```python
from build123d import *

# Parameters (mm, degrees)
SKETCH1_W           = 58
SKETCH1_H           = 23
BOSS_EXTRUDE1_DEPTH = 3
SKETCH2_W           = 3
SKETCH2_H           = 23
BOSS_EXTRUDE2_DEPTH = 1.5
SKETCH3_R           = 0.375
BOSS_EXTRUDE3_DEPTH = 5
LPATTERN1_COUNT     = 2
LPATTERN1_PITCH     = 50.8
SKETCH4_R           = 0.375
BOSS_EXTRUDE4_DEPTH = 5


with BuildPart() as part:
    # Sketch1 → Boss-Extrude1 (new body)
    with BuildSketch(Plane(origin=(0, 0, 0), x_dir=(1, 0, 0), z_dir=(0, 1, 0))):
        Rectangle(SKETCH1_W, SKETCH1_H)
    extrude(amount=BOSS_EXTRUDE1_DEPTH)

    # Sketch2 → Boss-Extrude2 (add)
    with BuildSketch(Plane.XZ):
        with Locations((-25.5, 0)):
            Rectangle(SKETCH2_W, SKETCH2_H)
    boss_extrude2 = extrude(amount=BOSS_EXTRUDE2_DEPTH)

    # Sketch3 → Boss-Extrude3 (add)
    with BuildSketch(Plane.XZ.offset(1.5)):
        with Locations(Location((-25.5, 8, 0), (0, 0, 270))):
            Circle(SKETCH3_R)
        with Locations(Location((-25.5, 0, 0), (0, 0, 270))):
            Circle(SKETCH3_R)
        with Locations(Location((-25.5, -8, 0), (0, 0, 270))):
            Circle(SKETCH3_R)
    extrude(amount=BOSS_EXTRUDE3_DEPTH)

    # LPattern1: Boss-Extrude2 ×2
    with Locations(*[(i * LPATTERN1_PITCH, 0, 0) for i in range(1, LPATTERN1_COUNT)]):
        add(boss_extrude2)

    # Sketch4 → Boss-Extrude4 (add)
    with BuildSketch(Plane.XZ.offset(1.5)):
        with Locations(Location((25.3, 8.5, 0), (0, 0, 270))):
            Circle(SKETCH4_R)
        with Locations(Location((25.3, 4.25, 0), (0, 0, 270))):
            Circle(SKETCH4_R)
        with Locations(Location((25.3, 0, 0), (0, 0, 270))):
            Circle(SKETCH4_R)
        with Locations(Location((25.3, -4.25, 0), (0, 0, 270))):
            Circle(SKETCH4_R)
        with Locations(Location((25.3, -8.5, 0), (0, 0, 270))):
            Circle(SKETCH4_R)
    extrude(amount=BOSS_EXTRUDE4_DEPTH)


solid = part.part
```
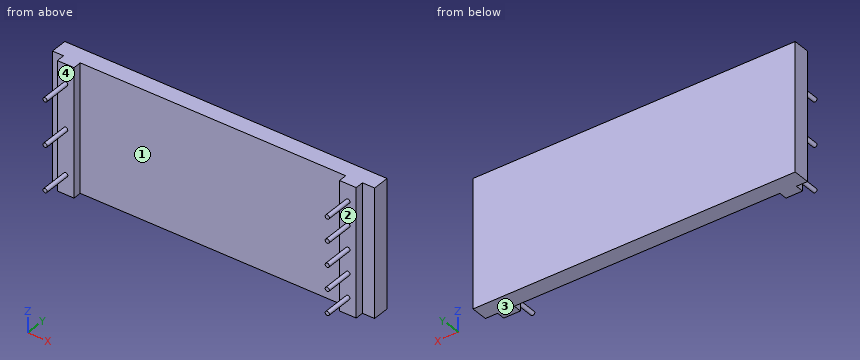
Work out the finished part from the listing and answer in its coordinate system (mm). Face numbers are marked on the shaded views. Round coordinates to 2 decimals unless told otherwise and drop trailing zeros. Loops run counter-clockwise (first coordinate to the right, second up) from the corner with the lowest first, then second, coordinate; pieces in that order, holes last. Notation, with made-up numbers: (25.25, 87) -> (47.25, 87) arc R36 ccw to (47.25, 121) -> close; hole circle Ø3 at (-13.5, -5.5). An arc over 180 degrees is marked (long way). Write each question's results on one line, items separated by ' | '. Start each with the question number.
1. Find the intervals of material crossed by probe 1 along X at (y, z) = (-3.25, 0) (3 decimals); probe 2 along X at (y, z) = (-1, 8.5); probe 3 along Y at (x, z) = (-14.5, -2.75), in increasing order. Write a range as from..to.
2. Given pin 1 Ø0.8 at (y, z) = (-1, -4) entering from +X; pin 2 Ø1.6 at (x, z) = (-28.5, -2.5) entering from -Y; pin 3 Ø3 at (y, z) = (-4, -3.5) entering from +X (3 decimals), each flat-ended and moving along its own axis, determine where each tip first touches the part or whether it passes through.
3. Section C-C (x = -16.5) is taken. Determine the outline of the cut face in (y, z).
4. For a pull along Z with two mould halves and no side action, classify the marked faces 1, 2, 3 and 4 as +Z half, -Z half, draft (parallel to the pull), parting line (faces both ways), or undercut.
5. Section B-B (z = -1) is taken. Determine the outline of the cut face in (x, y).
6. Section A-A (y = -5.5) is taken. Determine the outline of the cut face in (x, z) (3 decimals), plus the area to 3 significant figures.
Evaluation:
1) probe 1: x = -25.875..-25.125, 24.925..25.675 | probe 2: x = -27..-24, 23.8..26.8 | probe 3: y = 0..3
2) pin 1: stops at x = 26.8 | pin 2: stops at y = 0 | pin 3: stops at x = 25.675
3) outline: (0, -11.5) -> (3, -11.5) -> (3, 11.5) -> (0, 11.5) -> close
4) face 1: draft | face 2: undercut | face 3: -Z half | face 4: undercut
5) outline: (-29, 0) -> (-27, 0) -> (-27, -1.5) -> (-24, -1.5) -> (-24, 0) -> (23.8, 0) -> (23.8, -1.5) -> (26.8, -1.5) -> (26.8, 0) -> (29, 0) -> (29, 3) -> (-29, 3) -> close
6) outline: circle Ø0.75 at (-25.5, -8); circle Ø0.75 at (-25.5, 0); circle Ø0.75 at (-25.5, 8); circle Ø0.75 at (25.3, -8.5); circle Ø0.75 at (25.3, -4.25); circle Ø0.75 at (25.3, 0); circle Ø0.75 at (25.3, 4.25); circle Ø0.75 at (25.3, 8.5) | area: 3.53 mm2
